```python
from build123d import *

# Parameters (mm, degrees)
F2_R     = 19.8501
F3_DEPTH = 5.55625
F5_DEPTH = 254


with BuildPart() as f1:
    # F0 (on Front) → F1 (revolve)
    with BuildSketch(Plane.XZ):
        Polygon((1.00091, 0), (0, 0), (-2.445169, 0), (-6.818129, 12.7), (-11.137133, 12.7), (-11.137133, 10.324578), (-9.085405, 10.324578), (-8.059541, 0), (-8.059541, -16.51), (7.999178, -16.51), (7.999178, 0), (7.999178, 12.7), (5.373871, 12.7), align=None)
    revolve(axis=Axis((-0.030182, 0, -16.51), (1, 0, 0)))

    # F2 (on face) → F3 (join)
    with BuildSketch(Plane.YZ.offset(7.999178)):
        with Locations((0, -16.51)):
            Circle(F2_R)
    extrude(amount=F3_DEPTH)

    # F4 (on face) → F5 (cut)
    with BuildSketch(Plane.YZ.offset(13.555428)):
        with BuildLine():
            Line((-2.197634, -5.575972), (-2.197634, -9.778679))
            ThreePointArc((-2.197634, -9.778679), (-0.206109, -25.187333), (2.590266, -9.904236))
            Line((2.590266, -9.904236), (2.590266, -5.575972))
            Line((2.590266, -5.575972), (-2.197634, -5.575972))
        make_face()
    extrude(amount=-F5_DEPTH, mode=Mode.SUBTRACT)


solid = f1.part
```
Verification items for the finished model (mm, model axes). A direction names the side the tool comes from. Give positions to 0.01 mm unless a question says otherwise; leave off trailing zeros. Write each loop counter-clockwise with the first axis right and the second up, starting at its lowest first coordinate (ties: lowest second). Pieces come first, ordered by that corner, then holes. Notation, with made-up numbers: (11.25, -11.75) - (35.25, -11.75) arc R23 ccw to (35.25, 21.25) - close; hole circle Ø7 at (-39.5, 19.5). An arc over 180 degrees is marked (long way). Put each result on its own line as item: value.
Q1. Section check B-B on z = -16.51. Record the cut outline in (x, y), and give its area (3 significant figures).
Result:
outline: (-11.14, -29.21) - (-6.82, -29.21) - (-2.45, -16.51) - (1, -16.51) - (5.37, -29.21) - (8, -29.21) - (8, -19.85) - (13.56, -19.85) - (13.56, -7.82) - (-8.06, -7.82) - (-8.06, -16.51) - (-9.09, -26.83) - (-11.14, -26.83) - close; (-11.14, 26.83) - (-9.09, 26.83) - (-8.06, 16.51) - (-8.06, 7.82) - (13.56, 7.82) - (13.56, 19.85) - (8, 19.85) - (8, 29.21) - (5.37, 29.21) - (1, 16.51) - (-2.45, 16.51) - (-6.82, 29.21) - (-11.14, 29.21) - close
area: 647 mm2
Q2. Set-up check for faces 1 (the face through (7.999, 19, -23)), 2 (the face through (-0.746, -4.959, -0.762)), 3 (the face through (-11.137, 24, -4)), 4 (the face through (-10.097, -8.06, 9.085)), 5 (the face through (3, 0, -5.576)): record each of +Z, -Z, +X, -X, +Y, -Y from which the full face is reachable in a straight line by a thin tool's end or side.
Result:
face 1: +X
face 2: none
face 3: +Z, -Z, -X, +Y, -Y
face 4: -X
face 5: +X, -X
Q3. Section check A-A on y = 0. Record the cut outline in (x, z).
Result:
outline: (-11.14, -45.72) - (-6.82, -45.72) - (-2.45, -33.02) - (1, -33.02) - (5.37, -45.72) - (8, -45.72) - (8, -36.36) - (13.56, -36.36) - (13.56, -25.19) - (-8.06, -25.19) - (-8.06, -33.02) - (-9.09, -43.34) - (-11.14, -43.34) - close; (-11.14, 10.32) - (-9.09, 10.32) - (-8.06, 0) - (-8.06, -5.58) - (13.56, -5.58) - (13.56, 3.34) - (8, 3.34) - (8, 12.7) - (5.37, 12.7) - (1, 0) - (-2.45, 0) - (-6.82, 12.7) - (-11.14, 12.7) - close
Q4. Section check C-C on x = 12. Record the cut outline in (y, z), and give its area (3 significant figures).
Result:
outline: circle Ø39.7 at (0, -16.51); hole (-2.2, -9.78) arc R7.86 ccw (long way) to (2.59, -9.9) - (2.59, -5.58) - (-2.2, -5.58) - close
area: 1,020 mm2
Q5. Mould release check, pull along X, two halves, no side actions. Record for faces 6 (the face through (-2.72, -5.2, 0)), 7 (the face through (-8.06, 3, -9)), 8 (the face through (10.738, 18.933, -10.548)): released by +X, released by -X, zero draft, split by the parting line, or undercut.
Result:
face 6: undercut
face 7: released by -X
face 8: zero draft
Q6. Depth check by flat-ended pin: P1, Ø5, axis at x = -7, z = -12, coming from the -Y side; P2, Ø2, axis at y = -6.5, z = -11, coming from the -X side; P3, Ø10, axis at x = 7.5, z = -7, coming from the +Y side. Enter the tip coordinate at first touch or a pass-through.
Result:
P1: y = -29.14
P2: x = -8.06
P3: y = 28.86
Q7. Section check D-D on x = -5.75. Record the cut outline in (y, z).
Result:
outline: circle Ø52.22 at (0, -16.51); hole (-2.2, -9.78) arc R7.86 ccw (long way) to (2.59, -9.9) - (2.59, -5.58) - (-2.2, -5.58) - close
Q8. Scan lines: probe 1 along Z at (x, y) = (-0.75, 0); probe 2 along Y at (x, z) = (-9.6, -16.51); probe 3 along Z at (x, y) = (-10.7, 0). Record each from-to range of solid material in increasing order. Write a range as from..to.
Result:
probe 1: -33.02..-25.19, -5.58..0
probe 2: -29.21..-26.83, 26.83..29.21
probe 3: -45.72..-43.34, 10.32..12.7
